Read the model definition and answer for the solid it produces. Units are mm, in the model's axes. Coordinates: 2 decimals unless noted, no trailing zeros. Order: outer loops, then holes, each group sorted by start corner. A loop starts at its lowest first (then second) coordinate and runs counter-clockwise, first axis right, second up. Notation, with made-up numbers: (55.25, 9) -> (74.25, 9) arc R28 cw to (74.25, 43) -> close; hole circle Ø1 at (6.5, -25). An arc over 180 degrees is marked (long way). Use CSV: the item, a comma, the result in double quotes.
Autodesk Inventor part; units mm, degrees
ref_plane "YZ Plane" through (0, 0, 0) normal (1, 0, 0) x (0, 1, 0)
ref_plane "XZ Plane" through (0, 0, 0) normal (0, 1, 0) x (-1, 0, 0)
ref_plane "XY Plane" through (0, 0, 0) normal (0, 0, 1) x (1, 0, 0)
sketch "Sketch1" plane through (0, 0, 0) normal (0, 0, 1) x (1, 0, 0)
  line L0 (0, 0) -> (-7.4, 0)
  line L1 (-7.4, 0) -> (-7.4, 3)
  line L2 (-7.4, 3) -> (0, 3)
  line L3 (0, 3) -> (0, 0)
  line L4 (-7.4, 0) -> (-7.4, 0.8)
  line L5 (-7.4, 0.8) -> (-5.2, 3)
  dimension "d0" = 7.4
  dimension "d1" = 3
  dimension "d3" = 135
  dimension "d11" = 2.2
extrude "Extrusion1" add sketch "Sketch1" along normal blind 7.9 contours L0 L1 L5 L2 L3
sketch "Sketch2" plane through (-7.4, 0, 0) normal (0, -1, 0) x (1, 0, 0)
  line L0 (0, 0) -> (7.4, 0)
  line L1 (7.4, 0) -> (7.4, 7.9)
  line L2 (0, 7.9) -> (7.4, 7.9)
  line L3 (0, 0) -> (0, 7.9)
  circle A0 centre (3.7, 3.95) radius 1.5
  dimension "d6" = 3
extrude "Extrusion2" cut sketch "Sketch2" against normal blind 7.9 contours A0
sketch "Sketch3" plane through (-7.4, 0, 0) normal (0, -1, 0) x (1, 0, 0)
  point P0 (7.4, 0)
ref_plane "Work Plane1" through (-15.6286, 1.0607, 21.7368) normal (-0.7071, -0.7071, 0) x (0.7071, -0.7071, 0)
sketch "Sketch4" plane through (-15.6286, 1.0607, 21.7368) normal (-0.7071, -0.7071, 0) x (0.7071, -0.7071, 0)
  ellipse E0 centre (9.1848, -17.7868) end of major axis (9.1848, -16.2868) minor radius 1.0607 construction
  line L0 (6.5685, -21.7368) -> (11.8011, -21.7368)
  line L1 (11.8011, -21.7368) -> (11.8011, -13.8368)
  line L2 (6.5685, -13.8368) -> (11.8011, -13.8368)
  line L3 (6.5685, -21.7368) -> (6.5685, -13.8368)
  ellipse E1 centre (9.1848, -17.7868) end of major axis (9.1848, -16.2868) minor radius 1.0607 construction
  circle A0 centre (9.1848, -17.7868) radius 1.5 construction
  circle A1 centre (8.2455, -17.7868) radius 1.5374
extrude "Extrusion3" cut sketch "Sketch4" against normal through all contours A1
properties part number "00_KES400_DichroicMirror" material "PMMA Plastic"
Item 1: Each of these flat-tipped pins is pushed along its axis until it touches: P1, Ø1.5, axis at x = -6.5, y = 2.5, coming from the +Z side; P2, Ø1, axis at x = -5, z = 4.5, coming from the -Y side; P3, Ø2.5, axis at x = -3.7, z = 3.95, coming from the -Y side. Where does it stop, or does it pass through?
Return value:
P1,"stops at z = 7.9"
P2,"stops at y = 1.43"
P3,"passes through"
Item 2: Straight lines are drawn through the part: line 1 along Z through (x, y) = (-3.7, 0.45); line 2 along X through (y, z) = (2.3, 5.25); line 3 along Z through (x, y) = (-6, 0.75). For each, find the intervals that lie inside material, in ascending order.
Return value:
line 1,"z = 0 to 2.45, 5.45 to 7.9"
line 2,"x = -5.9 to -4.45, -1.57 to 0"
line 3,"z = 0 to 3.01, 4.89 to 7.9"
Item 3: The mould has two halves that part along Z. Classify faces 1 (the flat face through (-6.3, 1.9, 3.9)), 2 (the cylindrical face through (-5.2, 2.5, 4)), 3 (the flat face through (-4, 2, 7.9)): +Z half, -Z half, draft (parallel to the pull), parting line (faces both ways), or undercut.
Return value:
face 1,"draft"
face 2,"undercut"
face 3,"+Z half"
Item 4: Find section A-A, the plane z = 1.5. Give the vertices of the cut face in (x, y).
Return value:
outline,"(-7.4, 0) -> (0, 0) -> (0, 3) -> (-5.2, 3) -> (-7.4, 0.8) -> close"
